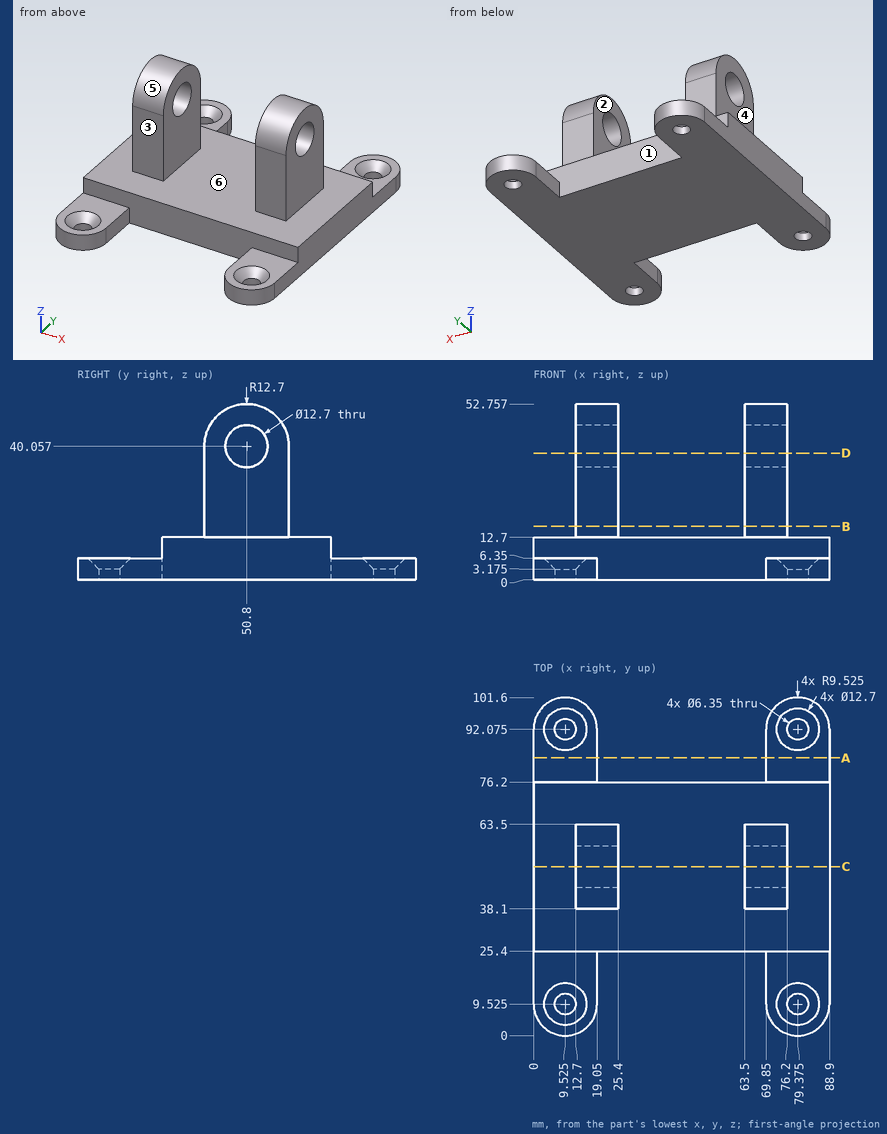
Study the drawing (mm; zero at the part's minimum x, y, z) and answer. A direction names the side the tool comes from. Give positions to 0.01 mm unless a question says otherwise; leave off trailing zeros. Write each loop counter-clockwise with the first axis right and the second up, starting at its lowest first coordinate (ties: lowest second). Pieces come first, ordered by that corner, then holes.
(1) Flat-ended cylindrical pins translate along their axes: pin 1 Ø7.5 at (x, y) = (9.525, 92.075) entering from +Z; pin 2 Ø5 at (y, z) = (80.5, 9.5) entering from -X; pin 3 Ø12 at (x, z) = (69.5, 43.5) entering from -Y; pin 4 Ø15 at (x, y) = (11.5, 91) entering from +Z. Find the tip coordinate at first contact, or state that the pin passes through.
Final values:
pin 1: stops at z = 3.75
pin 2: passes through
pin 3: stops at y = 38.1
pin 4: stops at z = 6.35
(2) The mould has two halves that part along X. Classify the marked faces 4, 5 and 6: pulls with the +X half, pulls with the -X half, needs draft (parallel to the pull), parting line crosses it, or undercut.
Final values:
face 4: pulls with the -X half
face 5: needs draft
face 6: undercut
(3) Which of the six approach directions +Z, -Z, +X, -X, +Y, -Y give full straight-line access (tool end or side, diameter ignored) to the marked faces 1, 2 and 3?
Final values:
face 1: +Z, +Y
face 2: +Z, +Y, -Y
face 3: +Z, +X, -X, -Y
(4) Straight lines are drawn through the part: line 1 (X direction, y = 96, z = 5.5); line 2 (X direction, y = 51.5, z = 16); line 3 (Z direction, x = 11, y = 28). For each, find the intervals that lie inside material, in ascending order.
Final values:
line 1: x = 0.85 to 5.67, 13.38 to 18.2, 70.7 to 75.52, 83.23 to 88.05
line 2: x = 12.7 to 25.4, 63.5 to 76.2
line 3: z = 0 to 12.7
(5) The part is cut by section C-C on y = 50.8. Write down the section's boundary in (x, z), plus the area to 3 significant figures.
Final values:
outline: (0, 0) - (88.9, 0) - (88.9, 12.7) - (76.2, 12.7) - (76.2, 33.71) - (63.5, 33.71) - (63.5, 12.7) - (25.4, 12.7) - (25.4, 33.71) - (12.7, 33.71) - (12.7, 12.7) - (0, 12.7) - close; (12.7, 46.41) - (25.4, 46.41) - (25.4, 52.76) - (12.7, 52.76) - close; (63.5, 46.41) - (76.2, 46.41) - (76.2, 52.76) - (63.5, 52.76) - close
area: 1,820 mm2
(6) The part is cut by section D-D on z = 38. Write down the section's boundary in (x, y), plus the area to 3 significant figures.
Final values:
outline: (12.7, 38.1) - (25.4, 38.1) - (25.4, 44.79) - (12.7, 44.79) - close; (12.7, 56.81) - (25.4, 56.81) - (25.4, 63.5) - (12.7, 63.5) - close; (63.5, 38.1) - (76.2, 38.1) - (76.2, 44.79) - (63.5, 44.79) - close; (63.5, 56.81) - (76.2, 56.81) - (76.2, 63.5) - (63.5, 63.5) - close
area: 340 mm2
(7) The part is cut by section B-B on z = 16. Write down the section's boundary in (x, y), plus the area to 3 significant figures.
Final values:
outline: (12.7, 38.1) - (25.4, 38.1) - (25.4, 63.5) - (12.7, 63.5) - close; (63.5, 38.1) - (76.2, 38.1) - (76.2, 63.5) - (63.5, 63.5) - close
area: 645 mm2
(8) The part is cut by section A-A on y = 83.5. Write down the section's boundary in (x, z).
Final values:
outline: (0, 0) - (19.05, 0) - (19.05, 6.35) - (0, 6.35) - close; (69.85, 0) - (88.9, 0) - (88.9, 6.35) - (69.85, 6.35) - close
